```python
from build123d import *

# Parameters (mm, degrees)
ESQUISSE1_W             = 50
ESQUISSE1_H             = 45
BOSS_EXTRU_1_DEPTH      = 3
ESQUISSE2_W             = 10
ESQUISSE2_H             = 3
ENL_V_MAT_EXTRU_1_DEPTH = 10
ESQUISSE3_W             = 15
ESQUISSE3_H             = 10
ENL_V_MAT_EXTRU_2_DEPTH = 10
ESQUISSE4_W             = 10
ESQUISSE4_H             = 3
ENL_V_MAT_EXTRU_3_DEPTH = 10


with BuildPart() as part:
    # Esquisse1 → Boss.-Extru.1 (new body)
    with BuildSketch(Plane.XY):
        with Locations((25, 22.5)):
            Rectangle(ESQUISSE1_W, ESQUISSE1_H)
    extrude(amount=BOSS_EXTRU_1_DEPTH)

    # Esquisse2 → Enlèv. mat.-Extru.1 (cut)
    with BuildSketch(Plane.XY.offset(3)):
        with Locations((15, 1.5)):
            Rectangle(ESQUISSE2_W, ESQUISSE2_H)
        with Locations((35, 1.5)):
            Rectangle(ESQUISSE2_W, ESQUISSE2_H)
    extrude(amount=-ENL_V_MAT_EXTRU_1_DEPTH, mode=Mode.SUBTRACT)

    # Esquisse3 → Enlèv. mat.-Extru.2 (cut)
    with BuildSketch(Plane.XY.offset(3)):
        with Locations((35, 30)):
            Rectangle(ESQUISSE3_W, ESQUISSE3_H)
        with Locations((15, 30)):
            Rectangle(ESQUISSE3_W, ESQUISSE3_H)
        with Locations((35, 15)):
            Rectangle(ESQUISSE3_W, ESQUISSE3_H)
        with Locations((15, 15)):
            Rectangle(ESQUISSE3_W, ESQUISSE3_H)
    extrude(amount=-ENL_V_MAT_EXTRU_2_DEPTH, mode=Mode.SUBTRACT)

    # Esquisse4 → Enlèv. mat.-Extru.3 (cut)
    with BuildSketch(Plane.XY.offset(3)):
        with Locations((15, 43.5)):
            Rectangle(ESQUISSE4_W, ESQUISSE4_H)
        with Locations((35, 43.5)):
            Rectangle(ESQUISSE4_W, ESQUISSE4_H)
    extrude(amount=-ENL_V_MAT_EXTRU_3_DEPTH, mode=Mode.SUBTRACT)


solid = part.part
```
For this review, take the finished solid that the model builds, in its own axes (mm). A direction names the side the tool comes from. Round coordinates to 2 decimals unless told otherwise and drop trailing zeros. Write each loop counter-clockwise with the first axis right and the second up, starting at its lowest first coordinate (ties: lowest second). Pieces come first, ordered by that corner, then holes. Notation, with made-up numbers: M 59,86 L 113,86 A14 cw 113,91 Z; hole C -24,20 d5. An arc over 180 degrees is marked long. One line per item, written item: value. Start each with the question number.
(1) Machinability: for faces 4 (the flat face through (35, 42, 2)), 5 (the flat face through (40, 1, 2)), 6 (the flat face through (15, 25, 2)), which of the approach directions +Z, -Z, +X, -X, +Y, -Y give a long, thin tool a straight path to every point of the face, cutting with its end or side? Answer none if there is none.
(2) The part is to be moulded in two halves that separate along X. For faces 1 (the flat face through (45, 45, 1)), 2 (the flat face through (40, 43, 2)), 3 (the flat face through (15, 42, 2)), say which applies: released by +X, released by -X, zero draft, split by the parting line, or undercut.
(3) Wall thickness on line 1 (Y direction, x = 38.5, z = 1.45); line 2 (X direction, y = 43.5, z = 0.5); line 3 (X direction, y = 17, z = 0.7): over which ranges is each line inside the solid? List them lowest first.
(4) We need section C-C (z = 2.1). Count the separate pieces of the cut face and the enclosed holes in it, and give its area (3 significant figures).
(5) We need section A-A (x = 41). Give the boundary of the cut face in (y, z), and give its area (3 significant figures).
(6) We need section B-B (y = 15). Give the boundary of the cut face in (x, z).
(7) Insertion check: pin 1 (0.9 mm diameter, centred on x = 17, z = 1, fed in from +Y); pin 2 (0.9 mm diameter, centred on x = 35.5, z = 1.5, fed in from -Y). Each pin has a flat end and moves straight along its axis. Give the tip position at first contact, or say it passes through.
Result:
1. face 4: +Z, -Z, +Y
1. face 5: +Z, -Z, -Y
1. face 6: +Z, -Z
2. face 1: zero draft
2. face 2: undercut
2. face 3: undercut
3. line 1: 3 to 10, 20 to 25, 35 to 42
3. line 2: 0 to 10, 20 to 30, 40 to 50
3. line 3: 0 to 7.5, 22.5 to 27.5, 42.5 to 50
4. separate pieces: 1
4. enclosed holes: 4
4. area: 1,530 mm²
5. outline: M 0,0 L 10,0 L 10,3 L 0,3 Z; M 20,0 L 25,0 L 25,3 L 20,3 Z; M 35,0 L 45,0 L 45,3 L 35,3 Z
5. area: 75.0 mm²
6. outline: M 0,0 L 7.5,0 L 7.5,3 L 0,3 Z; M 22.5,0 L 27.5,0 L 27.5,3 L 22.5,3 Z; M 42.5,0 L 50,0 L 50,3 L 42.5,3 Z
7. pin 1: y = 42
7. pin 2: y = 3
